Autodesk Inventor part; units mm, degrees
ref_plane "YZ Plane" through (0, 0, 0) normal (1, 0, 0) x (0, 1, 0)
ref_plane "XZ Plane" through (0, 0, 0) normal (0, 1, 0) x (-1, 0, 0)
ref_plane "XY Plane" through (0, 0, 0) normal (0, 0, 1) x (1, 0, 0)
sketch "Sketch5" plane through (0, 0, 0) normal (0, 1, 0) x (-1, 0, 0)
  line L0 (-37.5, -7.5) -> (37.5, -7.5)
  line L1 (37.5, -7.5) -> (37.5, 7.5)
  line L2 (37.5, 7.5) -> (-37.5, 7.5)
  line L3 (-37.5, 7.5) -> (-37.5, -7.5)
  line L4 (-37.5, -7.5) -> (37.5, 7.5) construction
  line L5 (37.5, -7.5) -> (-37.5, 7.5) construction
  point P0 (0, 0)
  dimension "d6" = 75
  dimension "d7" = 15
extrude "Extrusion2" add sketch "Sketch5" along normal blind 100
sketch "Sketch36" plane through (0, 0, 0) normal (0, -1, 0) x (1, 0, 0)
  line L0 (-37.5, 7.5) -> (37.5, 7.5)
  line L1 (0, 7.5) -> (0, -2.5)
  point P0 (0, 0)
  dimension "d82" = 10
hole "Hole1" at (0, 0, -2.5) direction (0, 1, 0) diameter 6.4 depth 10 tip angle 118
sketch "Sketch37" plane through (37.5, 0, -7.5) normal (0, 0, -1) x (-1, 0, 0)
  line L0 (37.5, 0) -> (55, 0)
  line L1 (75, 0) -> (0, 0)
  line L2 (70, 0) -> (70, 95)
  line L3 (0, 100) -> (75, 100)
  line L4 (70, 0) -> (165, 0) construction
  line L5 (70, 95) -> (5, 95)
  line L6 (0, 0) -> (0, 100)
  line L7 (5, 95) -> (5, 0)
  line L8 (5, 0) -> (0, 0)
  line L9 (0, 100) -> (75, 100)
  line L10 (75, 100) -> (75, 0)
  line L11 (55, 0) -> (70, 95)
  line L12 (5, 95) -> (70, 95)
  line L13 (37.5, 0) -> (20, 0)
  line L14 (20, 0) -> (5, 95)
  dimension "d90" = 17.5
  dimension "d91" = 95
  dimension "d92" = 90
  dimension "d93" = 65
  dimension "d94" = 17.5
extrude "Extrusion11" add sketch "Sketch37" along normal blind 10 contours L1 L14 L5 L11 L0
sketch "Sketch38" plane through (37.5, 100, -7.5) normal (0, 0, -1) x (-1, 0, 0)
  line L0 (75, -100) -> (0, -100)
  line L1 (1.5, -100) -> (3.5, -100)
  line L2 (3.5, -100) -> (3.5, -1.5)
  line L3 (3.5, -1.5) -> (1.5, -1.5)
  line L4 (1.5, -1.5) -> (1.5, -100)
  line L5 (1.5, -1.5) -> (73.5, -1.5)
  line L6 (73.5, -1.5) -> (73.5, -3)
  line L7 (73.5, -3) -> (1.5, -3)
  line L8 (1.5, -3) -> (1.5, -1.5)
  line L9 (55, -100) -> (75, -100)
  line L10 (73.5, -1.5) -> (71.5, -1.5)
  line L11 (71.5, -1.5) -> (71.5, -100)
  line L12 (71.5, -100) -> (73.5, -100)
  line L13 (73.5, -100) -> (73.5, -1.5)
  point P0 (37.5, -100)
  dimension "d97" = 2
  dimension "d98" = 98.5
  dimension "d99" = 72
  dimension "d100" = 2
extrude "Extrusion12" cut sketch "Sketch38" against normal blind 5 contours L0 L11 L7 L13 | L7 L11 L5 L6 | L7 L2 L5 L11 | L0 L4 L7 L2 | L7 L4 L3 L2
sketch "Sketch39" plane through (-37.5, 0, 7.5) normal (0, 0, 1) x (1, 0, 0)
  line L0 (42.5, 55) -> (32.5, 55)
  line L1 (32.5, 55) -> (32.5, 45)
  line L2 (32.5, 45) -> (42.5, 45)
  line L3 (42.5, 45) -> (42.5, 55)
  line L4 (42.5, 55) -> (32.5, 45) construction
  line L5 (32.5, 55) -> (42.5, 45) construction
  point P0 (37.5, 0)
  point P1 (37.5, 50)
  dimension "d103" = 10
  dimension "d104" = 10
extrude "Extrusion13" cut sketch "Sketch39" against normal blind 10
sketch "Sketch43" plane through (0, 0, 0) normal (0, -1, 0) x (1, 0, 0)
  line L0 (17.5, -7.5) -> (17.5, -17.5)
  line L1 (17.5, -17.5) -> (12.5, -17.5)
  line L2 (12.5, -17.5) -> (12.5, -12.5)
  line L3 (12.5, -12.5) -> (17.5, -12.5)
  line L4 (17.5, -12.5) -> (17.5, -17.5)
  line L5 (12.5, -12.5) -> (7.5, -12.5)
  line L6 (7.5, -12.5) -> (7.5, -7.5)
  line L7 (7.5, -7.5) -> (12.5, -7.5)
  line L8 (12.5, -7.5) -> (12.5, -12.5)
  point P0 (0, 0)
  dimension "d122" = 5
  dimension "d123" = 5
  dimension "d124" = 5
  dimension "d125" = 5
extrude "Extrusion16" add sketch "Sketch43" along normal blind 5 contours L5 L6 L7 L8
sketch "Sketch45" plane through (0, 0, 0) normal (0, -1, 0) x (1, 0, 0)
  line L0 (-17.5, -7.5) -> (-17.5, -17.5)
  line L1 (-17.5, -17.5) -> (-12.5, -17.5)
  line L2 (-12.5, -17.5) -> (-12.5, -12.5)
  line L3 (-12.5, -12.5) -> (-17.5, -12.5)
  line L4 (-17.5, -12.5) -> (-17.5, -17.5)
  line L5 (-12.5, -12.5) -> (-7.5, -12.5)
  line L6 (-7.5, -12.5) -> (-7.5, -7.5)
  line L7 (-7.5, -7.5) -> (-12.5, -7.5)
  line L8 (-12.5, -7.5) -> (-12.5, -12.5)
  point P0 (0, 0)
  dimension "d128" = 5
  dimension "d129" = 5
  dimension "d130" = 5
  dimension "d131" = 5
extrude "Extrusion17" add sketch "Sketch45" along normal blind 5 contours L8 L7 L6 L5
sketch "Sketch48" plane through (0, 0, 0) normal (0, -1, 0) x (1, 0, 0)
  line L0 (-27.5, 7.5) -> (27.5, 7.5)
  line L1 (27.5, 7.5) -> (27.5, -7.5)
  line L2 (27.5, -7.5) -> (-27.5, -7.5)
  line L3 (-27.5, -7.5) -> (-27.5, 7.5)
  line L4 (-27.5, 7.5) -> (27.5, -7.5) construction
  line L5 (27.5, 7.5) -> (-27.5, -7.5) construction
  line L6 (0, -7.5) -> (27.5, -7.5)
  line L7 (27.5, -7.5) -> (27.5, 7.5)
  line L8 (27.5, 7.5) -> (0, 7.5)
  line L9 (0, 7.5) -> (0, -7.5)
  line L10 (13.75, -7.5) -> (27.5, -7.5)
  line L11 (27.5, -7.5) -> (27.5, 7.5)
  line L12 (27.5, 7.5) -> (13.75, 7.5)
  line L13 (13.75, 7.5) -> (13.75, -7.5)
  line L14 (20.625, -7.5) -> (27.5, -7.5)
  line L15 (27.5, -7.5) -> (27.5, 7.5)
  line L16 (27.5, 7.5) -> (20.625, 7.5)
  line L17 (20.625, 7.5) -> (20.625, -7.5)
  line L18 (18.125, 2.5) -> (23.125, 2.5)
  line L19 (23.125, 2.5) -> (23.125, -2.5)
  line L20 (23.125, -2.5) -> (18.125, -2.5)
  line L21 (18.125, -2.5) -> (18.125, 2.5)
  line L22 (18.125, 2.5) -> (23.125, -2.5) construction
  line L23 (23.125, 2.5) -> (18.125, -2.5) construction
  point P0 (0, 0)
  point P1 (20.625, 0)
  dimension "d145" = 55
  dimension "d146" = 15
  dimension "d147" = 5
  dimension "d148" = 5
extrude "Extrusion20" add sketch "Sketch48" along normal blind 5 contours L18 L19 L20 L17 | L17 L20 L21 L18
sketch "Sketch49" plane through (0, 0, 0) normal (0, -1, 0) x (1, 0, 0)
  line L0 (-27.5, 7.5) -> (27.5, 7.5)
  line L1 (27.5, 7.5) -> (27.5, -7.5)
  line L2 (27.5, -7.5) -> (-27.5, -7.5)
  line L3 (-27.5, -7.5) -> (-27.5, 7.5)
  line L4 (-27.5, 7.5) -> (27.5, -7.5) construction
  line L5 (27.5, 7.5) -> (-27.5, -7.5) construction
  line L6 (0, -7.5) -> (-27.5, -7.5)
  line L7 (-27.5, -7.5) -> (-27.5, 7.5)
  line L8 (-27.5, 7.5) -> (0, 7.5)
  line L9 (0, 7.5) -> (0, -7.5)
  line L10 (0, -7.5) -> (-27.5, -7.5)
  line L11 (-27.5, -7.5) -> (-27.5, 7.5)
  line L12 (-27.5, 7.5) -> (0, 7.5)
  line L13 (0, 7.5) -> (0, -7.5)
  line L14 (-13.75, -7.5) -> (-27.5, -7.5)
  line L15 (-27.5, -7.5) -> (-27.5, 7.5)
  line L16 (-27.5, 7.5) -> (-13.75, 7.5)
  line L17 (-13.75, 7.5) -> (-13.75, -7.5)
  line L18 (-20.625, -7.5) -> (-27.5, -7.5)
  line L19 (-27.5, -7.5) -> (-27.5, 7.5)
  line L20 (-27.5, 7.5) -> (-20.625, 7.5)
  line L21 (-20.625, 7.5) -> (-20.625, -7.5)
  line L22 (-23.125, 2.5) -> (-18.125, 2.5)
  line L23 (-18.125, 2.5) -> (-18.125, -2.5)
  line L24 (-18.125, -2.5) -> (-23.125, -2.5)
  line L25 (-23.125, -2.5) -> (-23.125, 2.5)
  line L26 (-23.125, 2.5) -> (-18.125, -2.5) construction
  line L27 (-18.125, 2.5) -> (-23.125, -2.5) construction
  point P0 (0, 0)
  point P1 (-20.625, 0)
  dimension "d151" = 55
  dimension "d152" = 15
  dimension "d153" = 5
  dimension "d154" = 5
extrude "Extrusion21" add sketch "Sketch49" along normal blind 5 contours L22 L23 L24 L21 | L21 L24 L25 L22
properties part number "tb3_start"
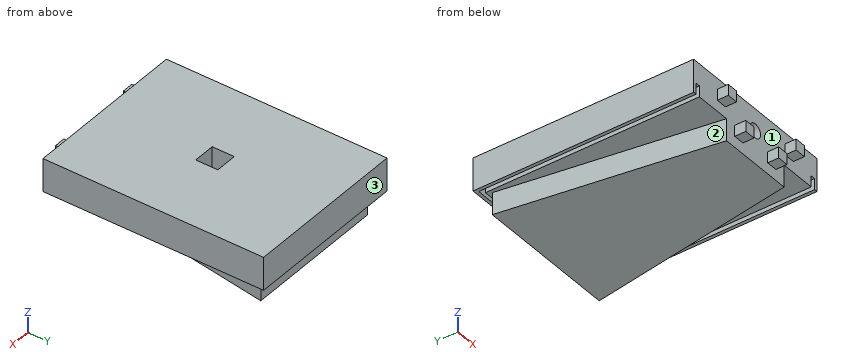
Build history of the part. All positions in model axes, mm. Face numbers are marked on the shaded views. Coordinates: 2 decimals unless noted, no trailing zeros. Write each loop counter-clockwise with the first axis right and the second up, starting at its lowest first coordinate (ties: lowest second). Pieces come first, ordered by that corner, then holes.
1. Drop flat-ended pins along their axis: pin 1 (5.5 mm diameter, centred on x = -20.5, y = -2.5, fed in from -Z); pin 2 (5.5 mm diameter, centred on y = -2, z = -10.5, fed in from -X); pin 3 (5.5 mm diameter, centred on y = -3, z = 1, fed in from +X) (3 decimals). Give the stop position or say it passes through.
Answer block:
pin 1: stops at z = -7.5
pin 2: stops at x = -17.62
pin 3: stops at x = 23.125
2. Band-saw the part on A-A, the plane y = 42.5. Give the cut face in (x, z).
Answer block:
outline: (-37.5, -7.5) - (-36, -7.5) - (-36, -2.5) - (-34, -2.5) - (-34, -7.5) - (-24.21, -7.5) - (-24.21, -17.5) - (24.21, -17.5) - (24.21, -7.5) - (34, -7.5) - (34, -2.5) - (36, -2.5) - (36, -7.5) - (37.5, -7.5) - (37.5, 7.5) - (-37.5, 7.5) - close
3. Drill centre lines: probe 1 along X at (y, z) = (64, -5.25); probe 2 along Z at (x, y) = (0, 3.5); probe 3 along Y at (x, z) = (1.5, -6). Where is each one in solid material? Low to high.
Answer block:
probe 1: x = -37.5 to -36, -34 to 34, 36 to 37.5
probe 2: z = -17.5 to -5.7, 0.7 to 7.5
probe 3: y = 0 to 97, 98.5 to 100
4. Band-saw the part on B-B, the plane x = 16. Give the cut face in (y, z), and give its area (3 significant figures).
Answer block:
outline: (0, -17.5) - (95, -17.5) - (95, -7.5) - (97, -7.5) - (97, -2.5) - (98.5, -2.5) - (98.5, -7.5) - (100, -7.5) - (100, 7.5) - (0, 7.5) - close
area: 2,440 mm2
5. Pull direction X, two halves, no side cores. Call the marked faces 1, 2 and 3: released by +X, released by -X, zero draft, split by the parting line, or undercut.
Answer block:
face 1: undercut
face 2: released by -X
face 3: zero draft
6. Band-saw the part on C-C, the plane y = 71. Give the cut face in (x, z), and give its area (3 significant figures).
Answer block:
outline: (-37.5, -7.5) - (-36, -7.5) - (-36, -2.5) - (-34, -2.5) - (-34, -7.5) - (-28.71, -7.5) - (-28.71, -17.5) - (28.71, -17.5) - (28.71, -7.5) - (34, -7.5) - (34, -2.5) - (36, -2.5) - (36, -7.5) - (37.5, -7.5) - (37.5, 7.5) - (-37.5, 7.5) - close
area: 1,680 mm2
